Autodesk Inventor part; units mm, degrees
ref_plane "YZ Plane" through (0, 0, 0) normal (1, 0, 0) x (0, 1, 0)
ref_plane "XZ Plane" through (0, 0, 0) normal (0, 1, 0) x (-1, 0, 0)
ref_plane "XY Plane" through (0, 0, 0) normal (0, 0, 1) x (1, 0, 0)
sketch "Sketch5" plane through (0, 0, 0) normal (1, 0, 0) x (0, 1, 0)
  line L0 (-38.1, 50.8) -> (38.1, 50.8)
  line L1 (50.8, 38.1) -> (50.8, -38.1)
  line L2 (38.1, -50.8) -> (-38.1, -50.8)
  line L3 (-50.8, -38.1) -> (-50.8, 38.1)
  line L4 (-50.8, 50.8) -> (50.8, -50.8) construction
  line L5 (50.8, 50.8) -> (-50.8, -50.8) construction
  arc A0 (50.8, 38.1) -> (38.1, 50.8) centre (38.1, 38.1) ccw
  arc A1 (38.1, -50.8) -> (50.8, -38.1) centre (38.1, -38.1) ccw
  arc A2 (-50.8, -38.1) -> (-38.1, -50.8) centre (-38.1, -38.1) ccw
  arc A3 (-38.1, 50.8) -> (-50.8, 38.1) centre (-38.1, 38.1) ccw
  line L6 (44.45, -38.1) -> (44.45, 38.1)
  arc A4 (44.45, 38.1) -> (38.1, 44.45) centre (38.1, 38.1) ccw
  line L7 (38.1, 44.45) -> (-38.1, 44.45)
  arc A5 (-38.1, 44.45) -> (-44.45, 38.1) centre (-38.1, 38.1) ccw
  line L8 (-44.45, 38.1) -> (-44.45, -38.1)
  arc A6 (-44.45, -38.1) -> (-38.1, -44.45) centre (-38.1, -38.1) ccw
  line L9 (-38.1, -44.45) -> (38.1, -44.45)
  arc A7 (38.1, -44.45) -> (44.45, -38.1) centre (38.1, -38.1) ccw
  point P0 (0, 0)
  dimension "d6" = 101.6
  dimension "d7" = 101.6
  dimension "d8" = 12.7
  dimension "d9" = 6.35
extrude "Extrusion4" add sketch "Sketch5" along normal mid plane 1111.25
properties part number "Front Hitch Model-2_Base Tube-1" material "SS304"
Check sheet for the modelled part. Datum: model origin and axes. Units: mm. A direction names the side the tool comes from. Round coordinates to 2 decimals unless told otherwise and drop trailing zeros. Write each loop counter-clockwise with the first axis right and the second up, starting at its lowest first coordinate (ties: lowest second). Pieces come first, ordered by that corner, then holes. Notation, with made-up numbers: M 32,10.25 L 54,10.25 A8 ccw 54,17.25 Z; hole C 12.25,64 d11. An arc over 180 degrees is marked long. Write item = value, one per line. Start each with the question number.
1. Tool access check on faces 4 (the flat face through (-8, 1, -50.8)), 5 (the flat face through (-8, 44.45, -1)). Record the directions out of +Z, -Z, +X, -X, +Y, -Y that give a thin tool (end or side, any length) a straight path to the whole face; none if there is none.
2. Release check for a two-part mould opening along Z. For faces 1 (the flat face through (-8, 1, 44.45)), 2 (the flat face through (-8, -1, 50.8)), 3 (the flat face through (-8, 50.8, 1)) record: pulls with the +Z half, pulls with the -Z half, needs draft (parallel to the pull), parting line crosses it, or undercut.
3. Section check C-C, the plane x = -342.5. Record the cut outline in (y, z).
4. Scan lines: line 1 (Z direction, x = 297, y = -26.5); line 2 (Y direction, x = 213, z = 39.5). Record each from-to range of solid material in increasing order. Write a range as [from, to].
5. Section check A-A, the plane y = -13. Record the cut outline in (x, z) (3 decimals).
Results found:
q1.face_4 = -Z, +X, -X, +Y, -Y
q1.face_5 = +X, -X
q2.face_1 = undercut
q2.face_2 = pulls with the +Z half
q2.face_3 = needs draft
q3.outline = M -50.8,-38.1 A12.7 ccw -38.1,-50.8 L 38.1,-50.8 A12.7 ccw 50.8,-38.1 L 50.8,38.1 A12.7 ccw 38.1,50.8 L -38.1,50.8 A12.7 ccw -50.8,38.1 Z; hole M -44.45,-38.1 A6.35 ccw -38.1,-44.45 L 38.1,-44.45 A6.35 ccw 44.45,-38.1 L 44.45,38.1 A6.35 ccw 38.1,44.45 L -38.1,44.45 A6.35 ccw -44.45,38.1 Z
q4.line_1 = [-50.8, -44.45], [44.45, 50.8]
q4.line_2 = [-50.72, -44.29], [44.29, 50.72]
q5.outline = M -555.625,-50.8 L 555.625,-50.8 L 555.625,-44.45 L -555.625,-44.45 Z; M -555.625,44.45 L 555.625,44.45 L 555.625,50.8 L -555.625,50.8 Z
